Geometry: see drawing. Coordinates: mm, zero at the bounding-box minimum. Give positions to 0.01 mm unless a question says otherwise; leave off trailing zeros. Order: outer loops, then holes, each group sorted by start corner. A loop starts at its lowest first (then second) coordinate and runs counter-clockwise, first axis right, second up. Notation, with made-up numbers: (18.25, 56) - (59.25, 56) arc R10 ccw to (59.25, 75) - close; hole circle Ø10 at (6, 52.5). An arc over 180 degrees is marked (long way). One line per item, written item: value.
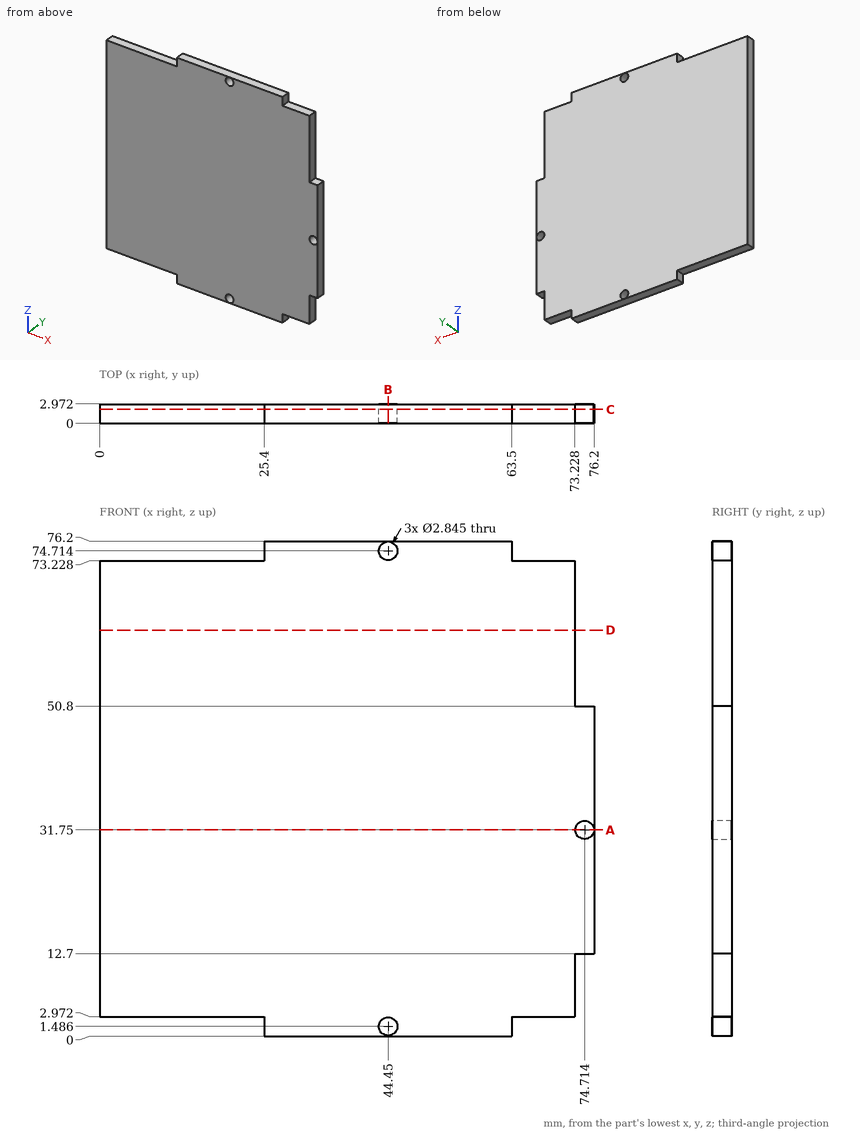
1) First-contact query: pin 1 (0.9 mm diameter, centred on x = 67.5, y = 1.5, fed in from -Z); pin 2 (0.9 mm diameter, centred on x = 75.5, y = 1, fed in from -Z). Flat tips, straight axial feed; report the tip coordinate or a pass-through.
Answers below:
pin 1: z = 2.97
pin 2: z = 12.7
2) Section C-C, the plane y = 2.15. Count the separate pieces of the cut face and the enclosed holes in it, then the cut area to 3 significant figures.
Answers below:
separate pieces: 1
enclosed holes: 3
area: 5,470 mm^2
3) Section D-D, the plane z = 62.5. Return loops of the section in (x, y).
Answers below:
outline: (0, 0) - (73.23, 0) - (73.23, 2.97) - (0, 2.97) - close
4) Material intervals for line 1 along X through (y, z) = (1.6, 66); line 2 along Z through (x, y) = (18.5, 1.55); line 3 along X through (y, z) = (2, 33) (1 decimal), sorted ascending.
Answers below:
line 1: 0 to 73.23
line 2: 2.97 to 73.23
line 3: 0 to 74, 75.4 to 76.2
5) Section A-A, the plane z = 31.75. Return loops of the section in (x, y), then the cut area to 3 significant figures.
Answers below:
outline: (0, 0) - (73.29, 0) - (73.29, 2.97) - (0, 2.97) - close; (76.14, 0) - (76.2, 0) - (76.2, 2.97) - (76.14, 2.97) - close
area: 218 mm^2
6) Section B-B, the plane x = 44.45. Return loops of the section in (y, z).
Answers below:
outline: (0, 0) - (2.97, 0) - (2.97, 0.06) - (0, 0.06) - close; (0, 2.91) - (2.97, 2.91) - (2.97, 73.29) - (0, 73.29) - close; (0, 76.14) - (2.97, 76.14) - (2.97, 76.2) - (0, 76.2) - close
